from build123d import *

# Parameters (mm, degrees)
F0_R     = 100
F1_DEPTH = 10
F3_R     = 6
F3_R_2   = 2.5
F4_DEPTH = 25
F5_D     = 2.5


with BuildPart() as f1:
    # F0 (on Front) → F1 (new body)
    with BuildSketch(Plane.XZ):
        Circle(F0_R)
    extrude(amount=F1_DEPTH)

    # F3 (on face) → F4 (join)
    with BuildSketch(Plane(origin=(0, 0, 0), x_dir=(-1, 0, 0), z_dir=(0, 1, 0))):
        Circle(F3_R)
        Circle(F3_R_2, mode=Mode.SUBTRACT)
    extrude(amount=F4_DEPTH)

    # F5 (through all)
    with Locations(Plane.XZ.offset(10)):
        with Locations((0, 0), (0, -65.783132)):
            Hole(F5_D / 2)


solid = f1.part
For this review, take the finished solid that the model builds, in its own axes (mm). A direction names the side the tool comes from. Round coordinates to 2 decimals unless told otherwise and drop trailing zeros. Loops run counter-clockwise (first coordinate to the right, second up) from the corner with the lowest first, then second, coordinate; pieces in that order, holes last. Notation, with made-up numbers: (-29.5, 4.5) - (19.5, 4.5) arc R26 cw to (19.5, 42.5) - close; hole circle Ø10 at (77.25, 47.5). An arc over 180 degrees is marked (long way). Put each result on its own line as item: value. Start each with the question number.
1. Consider section A-A on y = 7. State the section outline as (x, z) points, plus the area to 3 significant figures.
2. For probe 1 along Z at (x, y) = (0, -2.25); probe 2 along Z at (x, y) = (0, 13.75); probe 3 along Y at (x, z) = (-36, 0), list the stretches that pass through material, from the lowest coordinate up. Write a range as [from, to].
3. Consider section C-C on z = 60.5. State the section outline as (x, y) points.
4. For faces 4 (the flat face through (1, 0, 1)), 5 (the cylindrical face through (95.38, -4.93, 30.04)), list the 3-axis set-ups (+Z, -Z, +X, -X, +Y, -Y) from which the entire face can be reached by the end or side of a thin tool; tool diameter is ignored.
5. Mouldability with a two-part tool opening along X and no side actions: class faces 1 (the flat face through (-1, -10, 1)), 2 (the cylindrical face through (0.54, 12.32, -2.44)), 3 (the cylindrical face through (6, 12, 0)) as +X half, -X half, draft (parallel to the pull), parting line (faces both ways), or undercut.
6. Consider section B-B on x = -10.5. State the section outline as (y, z) points, plus the area to 3 significant figures.
7. Consider section D-D on y = -7. State the section outline as (x, z) points.
8. Insertion check: P1, Ø12, axis at y = -1, z = 76.5, coming from the -X side; P2, Ø3, axis at x = -26.5, z = -77.5, coming from the +Y side; P3, Ø4, axis at y = -4.5, z = -75.5, coming from the -X side. Each pin has a flat end and moves straight along its axis. Give the tip position at first contact, or say it passes through.
Result sheet:
1. outline: circle Ø12 at (0, 0); hole circle Ø5 at (0, 0)
1. area: 93.5 mm^2
2. probe 1: [-100, -67.03], [-64.53, -1.25], [1.25, 100]
2. probe 2: [-6, -2.5], [2.5, 6]
2. probe 3: [-10, 0]
3. outline: (-79.62, -10) - (79.62, -10) - (79.62, 0) - (-79.62, 0) - close
4. face 4: +Y
4. face 5: +Y, -Y
5. face 1: draft
5. face 2: undercut
5. face 3: parting line
6. outline: (-10, -99.45) - (0, -99.45) - (0, 99.45) - (-10, 99.45) - close
6. area: 1,990 mm^2
7. outline: circle Ø200 at (0, 0); hole circle Ø2.5 at (0, -65.78); hole circle Ø2.5 at (0, 0)
8. P1: x = -70.92
8. P2: y = 0
8. P3: x = -67.81
